Source: CAD feature listing. Evaluate the final solid. Frame: model axes, mm. A direction names the side the tool comes from. Give positions to 0.01 mm unless a question says otherwise; leave off trailing zeros. Order: outer loops, then holes, each group sorted by start corner. A loop starts at its lowest first (then second) coordinate and runs counter-clockwise, first axis right, second up. Notation, with made-up numbers: M 8.5,83 L 45.5,83 A23 cw 45.5,108 Z; hole C 86,-15.75 d1. An arc over 180 degrees is marked long. Answer in a Markdown table with one row per item. Add a question column.
(1) Pin query (flat end, axial travel): P1, Ø12, axis at x = 15.5, y = -263, coming from the +Z side; P2, Ø13, axis at y = -192.5, z = 44.5, coming from the +X side; P3, Ø12, axis at y = -192.5, z = 48.5, coming from the -X side. Return the tip coordinate at first contact, or that it passes through.
(2) Mould query, pull axis Y, two halves, no side actions, for faces 5 (the face through (30, 499, 34)), 6 (the face through (-10, 7, -16)), 7 (the face through (24.8, 489.5, -25)). Classes: pulls with the +Y half, pulls with the -Y half, needs draft (parallel to the pull), parting line crosses it, or undercut.
(3) Section query A-A, the plane z = 89.5. Return loops of the section in (x, y), plus the area to 3 significant figures.
(4) Material intervals for line 1 along Y through (x, z) = (57, 32.5); line 2 along Z through (x, y) = (45.5, -387.5); line 3 along Z through (x, y) = (2, 91.5), sorted ascending.
(5) Set-up query: faces 1 (the face through (0, -7, -33)), 2 (the face through (25, -491, -25)), 3 (the face through (10, -7, 48)), 4 (the face through (-8.4, -399.84, -44.72)). Return all of +Z, -Z, +X, -X, +Y, -Y with unobstructed straight access to the full face (end or side cutting, diameter ignored); none if empty.
from build123d import *

# Parameters (mm, degrees)
F1_DEPTH      = 489
F1_DEPTH_BACK = 489
F2_W          = 10
F2_H          = 100
F3_DEPTH      = 489
F3_DEPTH_BACK = 489
F5_DEPTH      = 10
F6_R          = 10
F7_R          = 8
F8_DEPTH      = 25
F9_T4_DEPTH   = 788.5183031967
F9_T9_DEPTH   = 788.5183031967
F13_R         = 8


# Not quite as in the source:
# - a fillet or chamfer that OpenCascade refuses, or shapes differently, is made with other operations: its cross-section is extruded or revolved along the edge and cut away or added
# - a pattern or mirror of a feature is missing from the dataset's text; its kind, count and spacing are read off the source's solid
# - a feature names something its author has since deleted; it is built from what else it names


with BuildPart() as f1:
    # F0 (on Front) → F1 (new body, two sides)
    with BuildSketch(Plane.XZ) as f1_sk:
        with BuildLine():
            Line((5, 75), (0, 75))
            Line((0, 75), (0, 0))
            Line((0, 0), (75, 0))
            Line((75, 0), (75, 5))
            ThreePointArc((75, 5), (73.5355339059, 8.5355339059), (70, 10))
            Line((70, 10), (26, 10))
            ThreePointArc((26, 10), (14.686291501, 14.686291501), (10, 26))
            Line((10, 26), (10, 70))
            ThreePointArc((10, 70), (8.5355339059, 73.5355339059), (5, 75))
        make_face()
    extrude(amount=F1_DEPTH)
    extrude(f1_sk.sketch, amount=-F1_DEPTH_BACK)

    # F2 (on Front) → F3 (join, two sides)
    with BuildSketch(Plane.XZ) as f3_sk:
        with Locations((-5, -15)):
            Rectangle(F2_W, F2_H)
    extrude(amount=F3_DEPTH)
    extrude(f3_sk.sketch, amount=-F3_DEPTH_BACK)

    # F4 (on face) → F5 (join)
    with BuildSketch(Plane(origin=(0, 489, 0), x_dir=(-1, 0, 0), z_dir=(0, 1, 0))):
        Polygon((-90, -25), (10, -25), (10, 125), (-8.5355339059, 125), (-90, -5), align=None)
    f5 = extrude(amount=F5_DEPTH)

    # F5_copies: F5 across plane
    add(f5.mirror(Plane(origin=(0, 0, 0), x_dir=(0, 0, -1), z_dir=(0, -1, 0))))

    # F6
    f6_edges = [f1.edges().sort_by_distance(p)[0] for p in [
        (8.535534, 494, 125),
        (90, 494, -5),
        (90, 494, -25),
        (-10, 494, 125),
        (-10, -494, 125),
        (8.535534, -494, 125),
        (90, -494, -25),
        (90, -494, -5),
    ]]
    fillet(f6_edges, radius=F6_R)

    # F7 (on face) → F8 (join)
    with BuildSketch(Plane(origin=(0, 499, 0), x_dir=(-1, 0, 0), z_dir=(0, 1, 0))):
        with Locations((-75, -10)):
            Circle(F7_R)
    f8 = extrude(amount=F8_DEPTH)

    # F8_copies: F8 across plane
    add(f8.mirror(Plane(origin=(0, 0, 0), x_dir=(0, 0, -1), z_dir=(0, -1, 0))))

    # F9: chamfer of 150 x 50 on 2 edges, made by hand


with BuildPart() as f9_tool2:
    # F9_s3 → F9_t4 (new body)
    with BuildSketch(Plane.YZ.offset(-399.2591515984)):
        Polygon((-489, -15), (-339, -65), (-489, -65), align=None)
    extrude(amount=F9_T4_DEPTH)

    split(bisect_by=Plane.XY.offset(-25), keep=Keep.BOTTOM)


with BuildPart() as f1_1:
    add(f1.part)

    # F9_t1: cut F9_tool2
    add(f9_tool2.part, mode=Mode.SUBTRACT)


with BuildPart() as f9_tool7:
    # F9_s8 → F9_t9 (new body)
    with BuildSketch(Plane.YZ.offset(-399.2591515984)):
        Polygon((339, -65), (489, -15), (489, -65), align=None)
    extrude(amount=F9_T9_DEPTH)

    split(bisect_by=Plane.XY.offset(-25), keep=Keep.BOTTOM)


with BuildPart() as f1_2:
    add(f1_1.part)

    # F9_t6: cut F9_tool7
    add(f9_tool7.part, mode=Mode.SUBTRACT)

    # F14: sweep along a path in F11
    with BuildLine(Plane(origin=(-5, 0, 0), x_dir=(0, -1, 0), z_dir=(-1, 0, 0))) as f14_path:
        Line((-434.5147456835, -41.0674455892), (-6.3245553203, -183.7975090436))
        ThreePointArc((-6.3245553203, -183.7975090436), (0, -184.8238430826), (6.3245553203, -183.7975090436))
        Line((6.3245553203, -183.7975090436), (444.0904629777, -37.8755398245))
    # F13 (on line) → F14 (sweep)
    with BuildSketch(Plane(origin=(0, 378.7430374384, 126.2476791461), x_dir=(-1, 0, 0), z_dir=(0, 0.9486832981, 0.316227766))):
        with Locations((5, -176.365627053)):
            Circle(F13_R)
    sweep(path=f14_path.line)


solid = f1_2.part
Values follow:
| question | item | result |
|---|---|---|
| 1 | P1 | stops at z = 72.18 |
| 1 | P2 | stops at x = 10 |
| 1 | P3 | stops at x = 0 |
| 2 | face 5 | pulls with the +Y half |
| 2 | face 6 | undercut |
| 2 | face 7 | needs draft |
| 3 | outline | M -10,-499 L 30.78,-499 L 30.78,-489 L -10,-489 Z; M -10,489 L 30.78,489 L 30.78,499 L -10,499 Z |
| 3 | area | 816 mm² |
| 4 | line 1 | y = -499 to -489, 489 to 499 |
| 4 | line 2 | z = 0 to 10 |
| 4 | line 3 | z = -159.49 to -151.32, 0 to 75 |
| 5 | face 1 | +X |
| 5 | face 2 | -Z, +X, -X, -Y |
| 5 | face 3 | +Z, +X |
| 5 | face 4 | none |
